```python
from build123d import *

# Parameters (mm, degrees)
SKETCH1_R           = 3.175
BOSS_EXTRUDE1_DEPTH = 6.35
FILLET2_R           = 12.7
FILLET3_R           = 2.116666667


with BuildPart() as part:
    # Sketch1 → Boss-Extrude1 (new body)
    with BuildSketch(Plane(origin=(0, 0, 0), x_dir=(1, 0, 0), z_dir=(0, 1, 0))):
        Polygon((120.65, 138.369431979), (120.65, 12.7), (95.25, 12.7), (95.25, -12.7), (120.65, -12.7), (146.05, -12.7), (171.45, -12.7), (171.45, 12.7), (146.05, 12.7), (146.05, 138.369431979), align=None)
        with Locations(Location((107.95, 0, 0), (0, 0, 270))):
            Circle(SKETCH1_R, mode=Mode.SUBTRACT)
        with Locations(Location((158.75, 0, 0), (0, 0, 270))):
            Circle(SKETCH1_R, mode=Mode.SUBTRACT)
        with BuildLine():
            Line((130.175, 35.731024811), (130.175, 125.669431979))
            ThreePointArc((130.175, 125.669431979), (133.35, 128.844431979), (136.525, 125.669431979))
            Line((136.525, 125.669431979), (136.525, 35.731024811))
            ThreePointArc((136.525, 35.731024811), (133.35, 32.556024811), (130.175, 35.731024811))
        make_face(mode=Mode.SUBTRACT)
    extrude(amount=BOSS_EXTRUDE1_DEPTH)

    # Fillet2
    fillet2_edges = [part.edges().sort_by_distance(p)[0] for p in [
        (120.65, 3.175, -138.369431979),
        (146.05, 3.175, -138.369431979),
        (146.05, 3.175, -12.7),
        (171.45, 3.175, 12.7),
        (171.45, 3.175, -12.7),
        (95.25, 3.175, 12.7),
        (95.25, 3.175, -12.7),
        (120.65, 3.175, -12.7),
    ]]
    fillet(fillet2_edges, radius=FILLET2_R - 0.0001)  # a hair under: the kernel refuses the full size

    # Fillet3
    fillet3_edges = [part.edges().sort_by_distance(p)[0] for p in [
        (120.65, 0, -75.53471599),
        (120.65, 6.35, -75.53471599),
        (133.35, 0, 12.7),
        (146.05, 0, -75.53471599),
        (98.96971459, 0, -8.98028541),
        (98.96971459, 0, 8.98028541),
        (167.73028541, 0, -8.98028541),
        (167.73028541, 0, 8.98028541),
        (142.33028541, 0, -134.64971739),
        (124.36971459, 0, -134.64971739),
        (146.05, 6.35, -75.53471599),
        (133.35, 6.35, 12.7),
        (98.96971459, 6.35, -8.98028541),
        (98.96971459, 6.35, 8.98028541),
        (167.73028541, 6.35, -8.98028541),
        (167.73028541, 6.35, 8.98028541),
        (142.33028541, 6.35, -134.64971739),
        (124.36971459, 6.35, -134.64971739),
        (149.76971459, 0, -16.41971459),
        (149.76971459, 6.35, -16.41971459),
        (116.93028541, 0, -16.41971459),
        (116.93028541, 6.35, -16.41971459),
    ]]
    fillet(fillet3_edges, radius=FILLET3_R)


solid = part.part
```
The listing builds one solid part. Answer for the finished solid, in the listing's coordinates (mm). A direction names the side the tool comes from. Coordinates: 2 decimals unless noted, no trailing zeros. Loops run counter-clockwise (first coordinate to the right, second up) from the corner with the lowest first, then second, coordinate; pieces in that order, holes last. Notation, with made-up numbers: (33.5, 70) -> (86.5, 70) arc R28 cw to (86.5, 99) -> close; hole circle Ø8 at (42.5, -24.75). An arc over 180 degrees is marked (long way). Return JSON: item names as keys, results as strings. Group by question number.
(1) Determine the mould class of faces 1 (the flat face through (139, 6.35, -36)), 2 (the flat face through (130.175, 3, -80)), 3 (the cylindrical face through (167.63, 3.19, -9.08)), 4 (the cylindrical face through (99.07, 3.19, -9.08)) for opening direction X: released by +X, released by -X, zero draft, split by the parting line, or undercut.
(2) Which of the six approach directions +Z, -Z, +X, -X, +Y, -Y give full straight-line access (tool end or side, diameter ignored) to faces 5 (the cylindrical face through (142.23, 3.19, -134.75)), 6 (the cylindrical face through (133.42, 3.131, -32.557))?
(3) A cutting plane is placed at B-B on y = 1. Count the separate pieces of the cut face and the enclosed holes in it, and give its area (3 significant figures).
(4) Find the intervals of material crossed by probe 1 along X at (y, z) = (2.5, 0) (3 decimals); probe 2 along Z at (x, y) = (158.75, 2) (3 decimals); probe 3 along X at (y, z) = (0.5, -78) (3 decimals), in increasing order. Write a range as from..to.
(5) Given pin 1 Ø1.1 at (y, z) = (2.5, -76) entering from -X; pin 2 Ø3 at (x, y) = (151, 5.5) entering from +Z; pin 3 Ø1.7 at (y, z) = (3.5, -58) entering from +X, each flat-ended and moving along its own axis, determine where each tip first touches the part or whether it passes through.
(6) A cutting plane is placed at A-A on z = -112. Write down the section's boundary in (x, y) (3 decimals), and give its area (3 significant figures).
The answers:
{
 "1": {"face 1": "zero draft", "face 2": "undercut", "face 3": "released by +X", "face 4": "released by -X"},
 "2": {"face 5": "-Z, +X, +Y, -Y", "face 6": "+Y, -Y"},
 "3": {"separate pieces": "1", "enclosed holes": "3", "area": "4,190 mm^2"},
 "4": {"probe 1": "x = 95.25..104.775, 111.125..155.575, 161.925..171.45", "probe 2": "z = -12.697..-3.175, 3.175..12.697", "probe 3": "x = 121.4..130.175, 136.525..145.3"},
 "5": {"pin 1": "stops at x = 120.65", "pin 2": "stops at z = 12.7", "pin 3": "stops at x = 146.05"},
 "6": {"outline": "(120.65, 2.117) arc R2.117 ccw to (122.767, 0) -> (130.175, 0) -> (130.175, 6.35) -> (122.767, 6.35) arc R2.117 ccw to (120.65, 4.233) -> close; (136.525, 0) -> (143.933, 0) arc R2.117 ccw to (146.05, 2.117) -> (146.05, 4.233) arc R2.117 ccw to (143.933, 6.35) -> (136.525, 6.35) -> close", "area": "117 mm^2"}
}
